Geometry: final body of the model. Coordinates: model frame, mm. Face numbers are marked on the shaded views. A direction names the side the tool comes from. Give positions to 0.01 mm unless a question says otherwise; leave off trailing zeros. Order: outer loops, then holes, each group sorted by start corner. A loop starts at its lowest first (then second) coordinate and runs counter-clockwise, first axis right, second up. Notation, with made-up numbers: (31, 12.5) -> (62, 12.5) arc R7 ccw to (62, 21.5) -> close; hole circle Ø9 at (38.5, -30). An arc over 180 degrees is marked (long way). One line per item, written item: value. Start each with the question number.
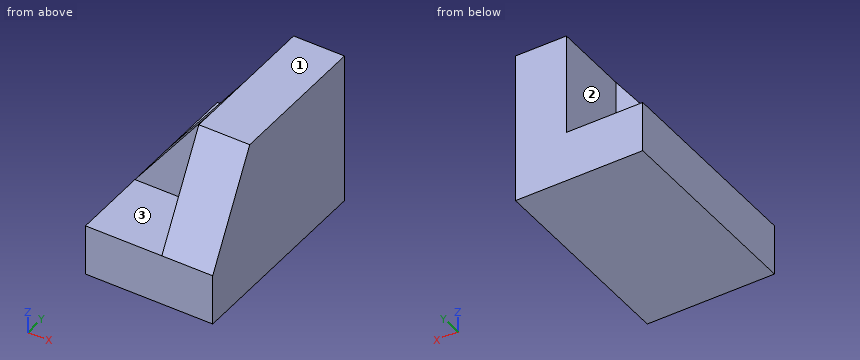
```python
from build123d import *

# Parameters (mm, degrees)
F1_DEPTH = 50.8
F3_DEPTH = 25.4
F4_W     = 12.7
F4_H     = 25.4
F5_DEPTH = 19.05
F7_DEPTH = 25.4


with BuildPart() as f1:
    # F0 (on Front) → F1 (new body)
    with BuildSketch(Plane.XZ):
        Polygon((0, 12.7), (0, 0), (31.75, 0), (31.75, 38.1), (19.05, 38.1), (19.05, 12.7), align=None)
    extrude(amount=F1_DEPTH)

    # F2 (on face) → F3 (cut)
    with BuildSketch(Plane(origin=(19.05, 0, 0), x_dir=(0, -1, 0), z_dir=(-1, 0, 0))):
        Polygon((36.5225, 38.1), (50.8, 12.7), (50.8, 38.1), align=None)
    extrude(amount=-F3_DEPTH, mode=Mode.SUBTRACT)

    # F4 (on face) → F5 (join)
    with BuildSketch(Plane(origin=(19.05, 0, 0), x_dir=(0, -1, 0), z_dir=(-1, 0, 0))):
        with Locations((25.4, 25.4)):
            Rectangle(F4_W, F4_H)
    extrude(amount=F5_DEPTH)

    # F6 (on face) → F7 (cut)
    with BuildSketch(Plane.XZ.offset(31.75)):
        Polygon((0, 12.7), (19.05, 38.1), (0, 38.1), align=None)
    extrude(amount=-F7_DEPTH, mode=Mode.SUBTRACT)


solid = f1.part
```
1. Cut plane C-C, the plane z = 29. Return loops of the section in (x, y) (3 decimals), then the cut area to 3 significant figures.
2. Cut plane A-A, the plane x = 15. Return loops of the section in (y, z).
3. Cut plane B-B, the plane y = -26.5. Return loops of the section in (x, z).
4. Material intervals for L1, parallel to X at y = -32, z = 14; L2, parallel to Z at x = 6, y = -39; L3, parallel to Y at x = 12.5, z = 16, sorted ascending. Write a range as [from, to].
5. Pin query (flat end, axial travel): P1, Ø21, axis at y = -44.5, z = 26, coming from the -X side; P2, Ø9.5, axis at x = 8, y = -46, coming from the +Z side; P3, Ø8, axis at x = 24.5, z = 22, coming from the -Y side. Return the tip coordinate at first contact, or that it passes through.
6. Access query for the marked faces 1, 2 and 3. Directions: +Z, -Z, +X, -X, +Y, -Y. A direction counts if a zero-diameter tool reaches every point of the face in a straight line with its end or side. Return the directions, or none.
7. Cut plane D-D, the plane y = -12. Return loops of the section in (x, z), then the cut area to 3 significant figures.
Answers follow:
1. outline: (12.225, -31.75) -> (19.05, -31.75) -> (19.05, -41.638) -> (31.75, -41.638) -> (31.75, 0) -> (19.05, 0) -> (19.05, -19.05) -> (12.225, -19.05) -> close
1. area: 615 mm²
2. outline: (-50.8, 0) -> (0, 0) -> (0, 12.7) -> (-19.05, 12.7) -> (-19.05, 32.7) -> (-31.75, 32.7) -> (-31.75, 12.7) -> (-50.8, 12.7) -> close
3. outline: (0, 0) -> (31.75, 0) -> (31.75, 38.1) -> (19.05, 38.1) -> (0, 12.7) -> close
4. L1: x = [19.05, 31.75]
4. L2: z = [0, 12.7]
4. L3: y = [-31.75, -19.05]
5. P1: stops at x = 19.05
5. P2: stops at z = 12.7
5. P3: stops at y = -47.82
6. face 1: +Z, +X, -X, +Y, -Y
6. face 2: +Z, -X, +Y
6. face 3: +Z, -X, -Y
7. outline: (0, 0) -> (31.75, 0) -> (31.75, 38.1) -> (19.05, 38.1) -> (19.05, 12.7) -> (0, 12.7) -> close
7. area: 726 mm²
